The model under review builds one solid part; all positions refer to its coordinate system, in mm. A direction names the side the tool comes from. Round coordinates to 2 decimals unless told otherwise and drop trailing zeros. Loops run counter-clockwise (first coordinate to the right, second up) from the corner with the lowest first, then second, coordinate; pieces in that order, holes last. Notation, with made-up numbers: (86, 50.25) -> (120, 50.25) arc R21 ccw to (120, 70.25) -> close; hole circle Ø7 at (86, 68.5). An arc over 180 degrees is marked (long way). Use CSV: the item, a comma, the result in double quotes. Start each with the question number.
```python
from build123d import *

# Parameters (mm, degrees)
BOSS_EXTRUDE1_DEPTH = 18
SHELL2_T            = -1


with BuildPart() as part:
    # Sketch1 → Boss-Extrude1 (new body)
    with BuildSketch(Plane(origin=(0, 0, 0), x_dir=(1, 0, 0), z_dir=(0, 1, 0))):
        Polygon((2.124611797, -2.924277266), (0, -9.463160018), (-2.124611797, -2.924277266), (-9, -2.924277266), (-3.437694101, 1.116974523), (-5.562305899, 7.655857275), (0, 3.614605486), (5.562305899, 7.655857275), (3.437694101, 1.116974523), (9, -2.924277266), align=None)
    extrude(amount=BOSS_EXTRUDE1_DEPTH)

    # Shell2
    shell2_openings = [part.faces().sort_by_distance(p)[0] for p in [
        (0, 18, 0),
    ]]
    offset(amount=SHELL2_T, openings=shell2_openings, kind=Kind.INTERSECTION)


solid = part.part
```
1. The part is to be moulded in two halves that separate along Z. For faces 5 (the face through (0.709, 9.381, 4.046)), 6 (the face through (-1, 0, 0)), 7 (the face through (6, 9, 2.924)), say which applies: pulls with the +Z half, pulls with the -Z half, needs draft (parallel to the pull), parting line crosses it, or undercut.
2. Take a section at C-C, the plane z = 0.25. Give the boundary of the cut face in (x, y).
3. For faces 1 (the face through (4, 9, 1.924)), 2 (the face through (2.742, 8.874, -5.607)), 3 (the face through (6.18, 8.874, 0.875)), 4 (the face through (-6.258, 8.874, 0.932)), list the 3-axis set-ups (+Z, -Z, +X, -X, +Y, -Y) from which the entire face can be reached by the end or side of a thin tool; tool diameter is ignored.
4. Clearance check with flat-ended pins moving along their axes: P1, Ø8, axis at y = 6.5, z = -2.5, coming from the -X side; P2, Ø2.5, axis at x = -4, y = 6, coming from the -Z side; P3, Ø4, axis at y = 8.5, z = 5, coming from the -X side. State where each tip first meets the part, or that it passes through.
5. Take a section at A-A, the plane y = 1.75. Give the boundary of the cut face in (x, z) (3 decimals), then the cut area to 3 significant figures.
6. Take a section at B-B, the plane x = -5. Give the boundary of the cut face in (y, z), then the cut area to 3 significant figures.
7. Take a section at D-D, the plane x = -3. Give the boundary of the cut face in (y, z).
8. For line 1 along X through (y, z) = (7.25, -4.5); line 2 along X through (y, z) = (10.25, -3); line 3 along X through (y, z) = (1.75, -6.25), list the stretches that pass through material, from the lowest coordinate up. Write a range as from..to.
Results:
1,face 5,"undercut"
1,face 6,"needs draft"
1,face 7,"pulls with the +Z half"
2,outline,"(-5.32, 0) -> (5.32, 0) -> (5.32, 18) -> (3.62, 18) -> (3.62, 1) -> (-3.62, 1) -> (-3.62, 18) -> (-5.32, 18) -> close"
3,face 1,"+Y"
3,face 2,"-Z, +Y, -Y"
3,face 3,"+X, +Y, -Y"
3,face 4,"-X, +Y, -Y"
4,P1,"x = -7.04"
4,P2,"z = -7.43"
4,P3,"x = -2.1"
5,outline,"(-9, 2.924) -> (-3.438, -1.117) -> (-5.562, -7.656) -> (0, -3.615) -> (5.562, -7.656) -> (3.438, -1.117) -> (9, 2.924) -> (2.125, 2.924) -> (0, 9.463) -> (-2.125, 2.924) -> close; hole (-5.922, 1.924) -> (-2.262, -0.735) -> (-3.66, -5.038) -> (0, -2.379) -> (3.66, -5.038) -> (2.262, -0.735) -> (5.922, 1.924) -> (1.398, 1.924) -> (0, 6.227) -> (-1.398, 1.924) -> close"
5,area,"57.0 mm²"
6,outline,"(0, -7.25) -> (18, -7.25) -> (18, -5.93) -> (0, -5.93) -> close; (0, 0.02) -> (18, 0.02) -> (18, 1.25) -> (1, 1.25) -> (1, 1.92) -> (18, 1.92) -> (18, 2.92) -> (0, 2.92) -> close"
6,area,"64.7 mm²"
7,outline,"(0, -5.79) -> (18, -5.79) -> (18, -4.56) -> (1, -4.56) -> (1, -3.01) -> (18, -3.01) -> (18, -0.2) -> (1, -0.2) -> (1, 1.92) -> (18, 1.92) -> (18, 2.92) -> (0, 2.92) -> close"
8,line 1,"-4.54..-3.49, -2.92..-1.22, 1.22..2.92, 3.49..4.54"
8,line 2,"-4.05..-3, -0.86..0.86, 3..4.05"
8,line 3,"-5.11..-3.63, 3.63..5.11"
